from build123d import *

# Parameters (mm, degrees)
SKETCH1_R               = 1.75
BOSS_EXTRUDE1_DEPTH     = 6
SKETCH2_R               = 1.25
CUT_EXTRUDE1_DEPTH      = 6.566489362
CUT_EXTRUDE1_DEPTH_BACK = 6.566489362


with BuildPart() as part:
    # Sketch1 → Boss-Extrude1 (new body)
    with BuildSketch(Plane.XY):
        with BuildLine():
            Line((-4.465425532, 5.566489362), (18.534574468, 5.566489362))
            ThreePointArc((18.534574468, 5.566489362), (24.10106383, 0), (18.534574468, -5.566489362))
            Line((18.534574468, -5.566489362), (-4.465425532, -5.566489362))
            ThreePointArc((-4.465425532, -5.566489362), (-10.031914894, 0), (-4.465425532, 5.566489362))
        make_face()
        with Locations((-4.465425532, 0)):
            Circle(SKETCH1_R, mode=Mode.SUBTRACT)
        with Locations((18.534574468, 0)):
            Circle(SKETCH1_R, mode=Mode.SUBTRACT)
    extrude(amount=BOSS_EXTRUDE1_DEPTH)

    # Sketch2 → Cut-Extrude1 (cut, two sides)
    with BuildSketch(Plane(origin=(0, 0, 0), x_dir=(1, 0, 0), z_dir=(0, 1, 0))) as cut_extrude1_sk:
        with Locations((18.534574468, -3)):
            Circle(SKETCH2_R)
        with Locations((-4.465425532, -3)):
            Circle(SKETCH2_R)
    extrude(amount=CUT_EXTRUDE1_DEPTH, mode=Mode.SUBTRACT)
    extrude(cut_extrude1_sk.sketch, amount=-CUT_EXTRUDE1_DEPTH_BACK, mode=Mode.SUBTRACT)


solid = part.part
The listing builds one solid part. Answer for the finished solid, in the listing's coordinates (mm). Coordinates: 2 decimals unless noted, no trailing zeros. Write each loop counter-clockwise with the first axis right and the second up, starting at its lowest first coordinate (ties: lowest second). Pieces come first, ordered by that corner, then holes. Notation, with made-up numbers: (84.5, 36) -> (105.5, 36) arc R8 ccw to (105.5, 51) -> close; hole circle Ø8 at (-15.5, 40.25). An arc over 180 degrees is marked (long way). One line per question, with ' | ' between items.
1. For a pull along Z with two mould halves and no side action, classify faces 1 (the flat face through (7, 5.566, 3)), 2 (the flat face through (7, 0, 0)), 3 (the cylindrical face through (-3.273, 3.365, 2.625)) as released by +Z, released by -Z, zero draft, split by the parting line, or undercut.
Verdict:
face 1: zero draft | face 2: released by -Z | face 3: undercut
2. Straight lines are drawn through the part: line 1 (X direction, y = 1, z = 1.75); line 2 (X direction, y = 2, z = 4); line 3 (Y direction, x = 20, z = 3). For each, find the intervals that lie inside material, in ascending order.
Verdict:
line 1: x = -9.94 to -5.9, -3.03 to 17.1, 19.97 to 24.01 | line 2: x = -9.66 to -5.22, -3.72 to 17.78, 19.28 to 23.73 | line 3: y = -5.37 to -0.96, 0.96 to 5.37
3. Section A-A (y = 0) is taken. Determine the outline of the cut face in (x, z).
Verdict:
outline: (-10.03, 0) -> (-6.22, 0) -> (-6.22, 6) -> (-10.03, 6) -> close; (-2.72, 0) -> (16.78, 0) -> (16.78, 6) -> (-2.72, 6) -> close; (20.28, 0) -> (24.1, 0) -> (24.1, 6) -> (20.28, 6) -> close
4. Given pin 1 Ø1.5 at (y, z) = (-0.5, 1) entering from -X; pin 2 Ø2 at (x, y) = (18.53, 0) entering from +Z, each flat-ended and moving along its own axis, determine where each tip first touches the part or whether it passes through.
Verdict:
pin 1: stops at x = -10.03 | pin 2: passes through
5. Section B-B (z = 3.5) is taken. Determine the outline of the cut face in (x, y), and give its area (3 significant figures).
Verdict:
outline: (-5.61, -5.45) -> (-5.61, -1.32) arc R1.75 cw to (-5.61, 1.32) -> (-5.61, 5.45) arc R5.57 ccw to start; (-3.32, -5.57) -> (17.39, -5.57) -> (17.39, -1.32) arc R1.75 cw to (17.39, 1.32) -> (17.39, 5.57) -> (-3.32, 5.57) -> (-3.32, 1.32) arc R1.75 cw to (-3.32, -1.32) -> close; (19.68, -5.45) arc R5.57 ccw to (19.68, 5.45) -> (19.68, 1.32) arc R1.75 cw to (19.68, -1.32) -> close | area: 298 mm^2
6. Section C-C (z = 1.25) is taken. Determine the outline of the cut face in (x, y), and give its area (3 significant figures).
Verdict:
outline: (-4.47, -5.57) -> (18.53, -5.57) arc R5.57 ccw to (18.53, 5.57) -> (-4.47, 5.57) arc R5.57 ccw to start; hole circle Ø3.5 at (-4.47, 0); hole circle Ø3.5 at (18.53, 0) | area: 334 mm^2
